Geometry: final body of the model. Coordinates: model frame, mm. A direction names the side the tool comes from. Coordinates: 2 decimals unless noted, no trailing zeros. Write each loop counter-clockwise with the first axis right and the second up, starting at its lowest first coordinate (ties: lowest second). Pieces come first, ordered by that corner, then holes.
from build123d import *

# Parameters (mm, degrees)
SKETCH_1_R          = 2.55
EXTRUDE_1_DEPTH     = 3
SKETCH_3_R          = 2.55
EXTRUDE_2_DEPTH     = 7
EXTRUDE_3_DEPTH     = 11
SKETCH_5_R          = 2.55
EXTRUDE_4_DEPTH     = 7
EXTRUDE_START       = 7
SKETCH_6_R          = 7
SKETCH_6_R_2        = 2.55
EXTRUDE_5_DEPTH     = 7
SKETCH_7_R          = 1.3
CUT_EXTRUDE_1_DEPTH = 5
SKETCH_8_R          = 1.3
CUT_EXTRUDE_2_DEPTH = 5
SKETCH_9_R          = 5
CUT_EXTRUDE_3_DEPTH = 1.5
CUT_EXTRUDE_4_REACH = 38.718
FILLET_1_R          = 2


with BuildPart() as part:
    # Эскиз1 → Бобышка-Вытянуть1 (new body)
    with BuildSketch(Plane(origin=(0, 0, 0), x_dir=(1, 0, 0), z_dir=(0, 1, 0))):
        with BuildLine():
            Line((8.8, 25), (-16.8, 25))
            Line((-16.8, 25), (-16.8, -3))
            ThreePointArc((-16.8, -3), (-16.214213562, -4.414213562), (-14.8, -5))
            Line((-14.8, -5), (-13.979301231, -5))
            ThreePointArc((-13.979301231, -5), (-12.565087669, -5.585786438), (-11.979301231, -7))
            Line((-11.979301231, -7), (-11.979301231, -17.343145751))
            ThreePointArc((-11.979301231, -17.343145751), (-9.736660544, -22.757359313), (-4.322446982, -25))
            Line((-4.322446982, -25), (16.8, -25))
            Line((16.8, -25), (16.8, 17))
            Line((16.8, 17), (8.8, 25))
        make_face()
        with Locations(Location((4.8, 3.5, 0), (0, 0, 270))):
            Circle(SKETCH_1_R, mode=Mode.SUBTRACT)
        with Locations(Location((-3.489533647, -13.352791034, 0), (0, 0, 270))):
            Circle(SKETCH_1_R, mode=Mode.SUBTRACT)
    extrude(amount=EXTRUDE_1_DEPTH)

    # Эскиз3 → Бобышка-Вытянуть2 (add)
    with BuildSketch(Plane(origin=(0, 3, 0), x_dir=(1, 0, 0), z_dir=(0, 1, 0))):
        with BuildLine():
            Line((8.8, 25), (-16.8, 25))
            Line((-16.8, 25), (-16.8, -2.352791034))
            Line((-16.8, -2.352791034), (-3.489533647, -2.352791034))
            ThreePointArc((-3.489533647, -2.352791034), (4.288640946, -5.574616441), (7.510466353, -13.352791034))
            Line((7.510466353, -13.352791034), (7.510466353, -25))
            Line((7.510466353, -25), (16.8, -25))
            Line((16.8, -25), (16.8, 17))
            Line((16.8, 17), (8.8, 25))
        make_face()
        with Locations(Location((4.8, 3.5, 0), (0, 0, 270))):
            Circle(SKETCH_3_R, mode=Mode.SUBTRACT)
    extrude(amount=EXTRUDE_2_DEPTH)

    # Эскиз4 → Бобышка-Вытянуть3 (add)
    with BuildSketch(Plane(origin=(0, 10, 0), x_dir=(1, 0, 0), z_dir=(0, 1, 0))):
        with BuildLine():
            Line((8.8, 25), (-16.8, 25))
            Line((-16.8, 25), (-16.8, 14.51476677))
            Line((-16.8, 14.51476677), (5.031765415, 14.51476677))
            ThreePointArc((5.031765415, 14.51476677), (13.930610034, 9.983309776), (15.5, 0.121233261))
            Line((15.5, 0.121233261), (15.5, -25))
            Line((15.5, -25), (16.8, -25))
            Line((16.8, -25), (16.8, 17))
            Line((16.8, 17), (8.8, 25))
        make_face()
    extrude(amount=EXTRUDE_3_DEPTH)

    # Эскиз5 → Бобышка-Вытянуть4 (add)
    with BuildSketch(Plane(origin=(0, 21, 0), x_dir=(1, 0, 0), z_dir=(0, 1, 0))):
        with BuildLine():
            Line((8.8, 25), (-16.8, 25))
            Line((-16.8, 25), (-16.8, -3))
            ThreePointArc((-16.8, -3), (-16.214213562, -4.414213562), (-14.8, -5))
            Line((-14.8, -5), (-13.979301231, -5))
            ThreePointArc((-13.979301231, -5), (-12.565087669, -5.585786438), (-11.979301231, -7))
            Line((-11.979301231, -7), (-11.979301231, -23))
            ThreePointArc((-11.979301231, -23), (-11.393514794, -24.414213562), (-9.979301231, -25))
            Line((-9.979301231, -25), (16.8, -25))
            Line((16.8, -25), (16.8, 17))
            Line((16.8, 17), (8.8, 25))
        make_face()
        with Locations(Location((4.8, 3.5, 0), (0, 0, 270))):
            Circle(SKETCH_5_R, mode=Mode.SUBTRACT)
        with Locations(Location((-3.489533647, -13.352791034, 0), (0, 0, 270))):
            Circle(SKETCH_5_R, mode=Mode.SUBTRACT)
    extrude(amount=EXTRUDE_4_DEPTH)

    # Эскиз6 → Бобышка-Вытянуть5 (add)
    with BuildSketch(Plane.XZ.offset(-21).offset(EXTRUDE_START)):
        with Locations(Location((-3.489533647, 13.352791034, 0), (0, 0, 90))):
            Circle(SKETCH_6_R)
        with Locations(Location((-3.489533647, 13.352791034, 0), (0, 0, 90))):
            Circle(SKETCH_6_R_2, mode=Mode.SUBTRACT)
    extrude(amount=-EXTRUDE_5_DEPTH)

    # Эскиз7 → Вырез-Вытянуть1 (cut)
    with BuildSketch(Plane(origin=(0, 0, -25), x_dir=(-1, 0, 0), z_dir=(0, 0, -1))):
        with Locations((4, 13.75)):
            Circle(SKETCH_7_R)
    extrude(amount=-CUT_EXTRUDE_1_DEPTH, mode=Mode.SUBTRACT)

    # Эскиз8 → Вырез-Вытянуть2 (cut)
    with BuildSketch(Plane(origin=(16.8, 0, 0), x_dir=(0, 0, -1), z_dir=(1, 0, 0))):
        with Locations((-4, 7)):
            Circle(SKETCH_8_R)
    extrude(amount=-CUT_EXTRUDE_2_DEPTH, mode=Mode.SUBTRACT)

    # Эскиз9 → Вырез-Вытянуть3 (cut)
    with BuildSketch(Plane.XZ):
        with Locations(Location((-3.489533647, 13.352791034, 0), (0, 0, 270))):
            Circle(SKETCH_9_R)
        with Locations(Location((4.8, -3.5, 0), (0, 0, 270))):
            Circle(SKETCH_9_R)
    extrude(amount=-CUT_EXTRUDE_3_DEPTH, mode=Mode.SUBTRACT)

    # Эскиз10 → Вырез-Вытянуть4 (cut, up to next)
    with BuildSketch(Plane.XZ.offset(-21), mode=Mode.PRIVATE) as cut_extrude_4_sk1:
        with BuildLine():
            Line((-4.322446982, 25), (-11.979301231, 25))
            Line((-11.979301231, 25), (-11.979301231, 17.343145751))
            ThreePointArc((-11.979301231, 17.343145751), (-9.736660544, 22.757359313), (-4.322446982, 25))
        make_face()
    cut_extrude_4_tool1 = extrude(cut_extrude_4_sk1.sketch, amount=-CUT_EXTRUDE_4_REACH, mode=Mode.PRIVATE) & part.part
    add(cut_extrude_4_tool1.solids().sort_by_distance((-10.269005, 21, 23.289704))[0], mode=Mode.SUBTRACT)

    # Скругление1
    fillet_1_edges = [part.edges().sort_by_distance(p)[0] for p in [
        (-3.489533647, 21, 6.352791034),
    ]]
    fillet(fillet_1_edges, radius=FILLET_1_R)


solid = part.part
Item 1: Pin query (flat end, axial travel): pin 1 (0.9 mm diameter, centred on x = -14.5, y = 1.5, fed in from +Z); pin 2 (2 mm diameter, centred on x = -11.5, y = 6, fed in from +Z); pin 3 (1.5 mm diameter, centred on y = 1.5, z = 10, fed in from -X); pin 4 (2 mm diameter, centred on x = 6, z = -3, fed in from -Y). Return the tip coordinate at first contact, or that it passes through.
Derived:
pin 1: stops at z = 5
pin 2: stops at z = 2.35
pin 3: stops at x = -11.98
pin 4: passes through
Item 2: Section C-C, the plane y = 9.25. Output: boundary loops of the cut face in (x, z), plus the area to 3 significant figures.
Derived:
outline: (-16.8, -25) - (8.8, -25) - (16.8, -17) - (16.8, 25) - (7.51, 25) - (7.51, 13.35) arc R11 cw to (-3.49, 2.35) - (-16.8, 2.35) - close; hole circle Ø5.1 at (4.8, -3.5)
area: 1,100 mm2
Item 3: Section B-B, the plane y = 18.25. Output: boundary loops of the cut face in (x, z), plus the area to 3 significant figures.
Derived:
outline: (-16.8, -25) - (8.8, -25) - (16.8, -17) - (16.8, 25) - (15.5, 25) - (15.5, -0.12) arc R11 cw to (5.03, -14.51) - (-16.8, -14.51) - close; circle Ø14 at (-3.49, 13.35); hole circle Ø5.1 at (-3.49, 13.35)
area: 524 mm2
Item 4: Set-up query: faces 4 (the flat face through (-2, 3, 11)), 5 (the cylindrical face through (-10.43, 16.51, 12.44)), 6 (the flat face through (-2, 1.5, 16)). Return all of +Z, -Z, +X, -X, +Y, -Y with unobstructed straight access to the full face (end or side cutting, diameter ignored); none if empty.
Derived:
face 4: +Z, -X
face 5: none
face 6: -Y
Item 5: Material intervals for probe 1 along Y at (x, z) = (13.7, 4); probe 2 along Y at (x, z) = (-13, -5); probe 3 along Y at (x, z) = (-4, 3.5), sorted ascending.
Derived:
probe 1: y = 0 to 5.7, 8.3 to 10, 21 to 28
probe 2: y = 0 to 10, 21 to 28
probe 3: y = 0 to 3, 21 to 28
Item 6: Section A-A, the plane y = 22. Output: boundary loops of the cut face in (x, z), plus the area to 3 significant figures.
Derived:
outline: (-16.8, -25) - (8.8, -25) - (16.8, -17) - (16.8, 25) - (-4.32, 25) arc R7.66 ccw to (-11.98, 17.34) - (-11.98, 7) arc R2 cw to (-13.98, 5) - (-14.8, 5) arc R2 ccw to (-16.8, 3) - close; hole circle Ø5.1 at (-3.49, 13.35); hole circle Ø5.1 at (4.8, -3.5)
area: 1,500 mm2
Item 7: Pull-direction query (Z, two-part tool) for faces 1 (the flat face through (8, 8, 25)), 2 (the flat face through (6, 1.5, -1)), 3 (the flat face through (0, 0, 0)); classes: released by +Z, released by -Z, zero draft, split by the parting line, or undercut.
Derived:
face 1: released by +Z
face 2: undercut
face 3: zero draft
